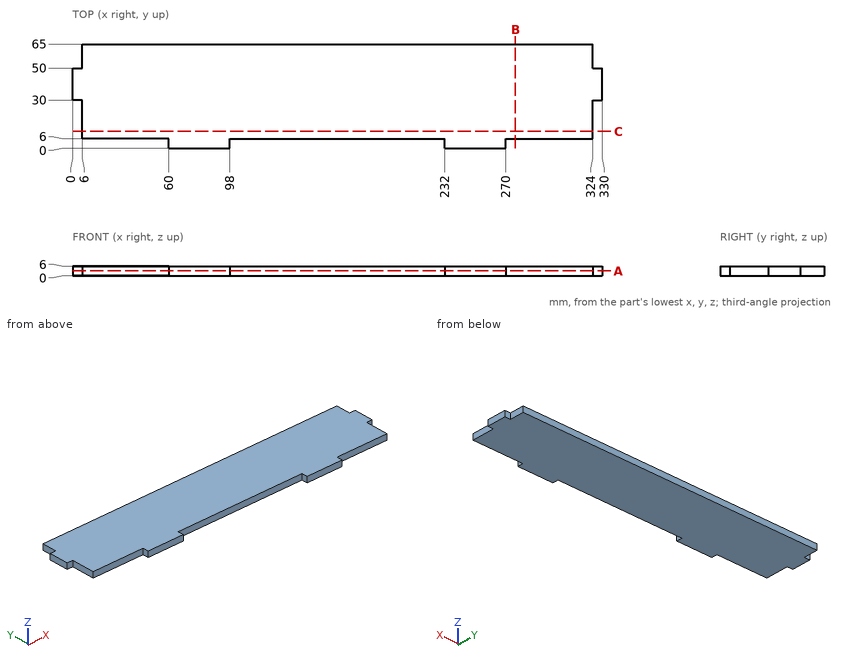
The drawing under review shows one solid part. Ordinate dimensions are in mm from its lowest x, y, z. Coordinates: 2 decimals unless noted, no trailing zeros. Order: outer loops, then holes, each group sorted by start corner. A loop starts at its lowest first (then second) coordinate and runs counter-clockwise, first axis right, second up. Notation, with made-up numbers: (46, 27.25) - (101, 27.25) arc R15 ccw to (101, 38.25) - close; hole circle Ø9 at (32.25, 86). An arc over 180 degrees is marked (long way). Put each result on its own line as item: value.
1) Take a section at A-A, the plane z = 3.15. Give the boundary of the cut face in (x, y), and give its area (3 significant figures).
Response values:
outline: (0, 30) - (6, 30) - (6, 6) - (60, 6) - (60, 0) - (98, 0) - (98, 6) - (232, 6) - (232, 0) - (270, 0) - (270, 6) - (324, 6) - (324, 30) - (330, 30) - (330, 50) - (324, 50) - (324, 65) - (6, 65) - (6, 50) - (0, 50) - close
area: 19,500 mm²
2) Take a section at B-B, the plane x = 276. Give the boundary of the cut face in (y, z).
Response values:
outline: (6, 0) - (65, 0) - (65, 6) - (6, 6) - close
3) Wall thickness on L1, parallel to X at y = 5, z = 2.05; L2, parallel to X at y = 62.5, z = 5.15; L3, parallel to Y at x = 201.5, z = 4.1: over which ranges is each line inside the solid? List them lowest first. Write a range as from..to.
Response values:
L1: x = 60..98, 232..270
L2: x = 6..324
L3: y = 6..65
4) Take a section at C-C, the plane y = 10.5. Give the boundary of the cut face in (x, z), and give its area (3 significant figures).
Response values:
outline: (6, 0) - (324, 0) - (324, 6) - (6, 6) - close
area: 1,910 mm²
5) Insertion check: P1, Ø3, axis at x = 118.5, z = 4.5, coming from the -Y side; P2, Ø3, axis at x = 327, z = 4, coming from the -Y side; P3, Ø12, axis at x = 238.5, y = 52.5, coming from the -Z side; P4, Ø3, axis at y = 58.5, z = 3.5, coming from the -X side. Each pin has a flat end and moves straight along its axis. Give the tip position at first contact, or say it passes through.
Response values:
P1: stops at y = 6
P2: stops at y = 30
P3: stops at z = 0
P4: stops at x = 6
